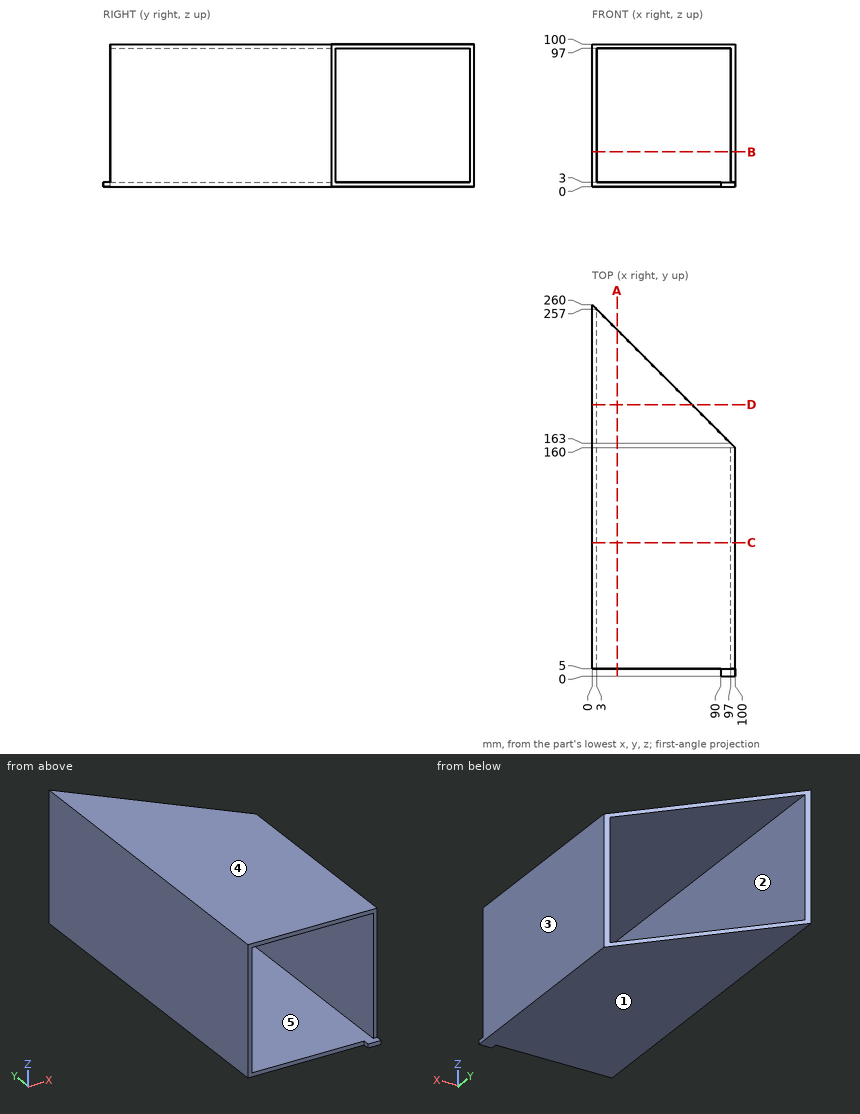
Here's the drawing with two shaded views (mm, measured from the low corner). I have some questions. A direction names the side the tool comes from. Give positions to 0.01 mm unless a question says otherwise; leave off trailing zeros. Order: outer loops, then holes, each group sorted by start corner. A loop starts at its lowest first (then second) coordinate and runs counter-clockwise, first axis right, second up.
Q1. Suppose I cut it at B-B, the plane z = 24.5. Write out the boundary of the cut face in (x, y).
Q2. Suppose I cut it at C-C, the plane y = 93.5. Write out the boundary of the cut face in (x, z), and give its area (3 significant figures).
Q3. For the marked faces 1 and 2, which set-ups out of +Z, -Z, +X, -X, +Y, -Y let a thin tool reach every point of the face, with its end or its side?
Q4. Suppose I cut it at D-D, the plane y = 190. Write out the boundary of the cut face in (x, z), and give its area (3 significant figures).
Q5. If I drill on line 1 along X through (y, z) = (90.5, 35.5); line 2 along X through (y, z) = (169, 17.5), over which ranges is the centre line in solid material (lowest first)?
Q6. Suppose I cut it at A-A, the plane x = 17.5. Write out the boundary of the cut face in (y, z), and give its area (4 significant figures).
Q7. I'm going to push flat-ended pins straight in: P1, Ø0.9, axis at y = 3, z = 2, coming from the -X side; P2, Ø2, axis at x = 31, y = 170, coming from the -Z side; P3, Ø1, axis at y = 177.5, z = 42.5, coming from the +X side. Where does each tip first touch, or does it pass through?
Q8. We'd pull the mould along Z, two halves only. Please class the marked faces 3, 4 and 5: +Z half, -Z half, draft (parallel to the pull), parting line (faces both ways), or undercut.
Solution:
1. outline: (0, 5) - (3, 5) - (3, 257) - (0, 260) - close; (97, 5) - (100, 5) - (100, 160) - (97, 163) - close
2. outline: (0, 0) - (100, 0) - (100, 100) - (0, 100) - close; hole (3, 3) - (97, 3) - (97, 97) - (3, 97) - close
2. area: 1,160 mm2
3. face 1: -Z, +X, -X, +Y, -Y
3. face 2: +Y, -Y
4. outline: (0, 0) - (70, 0) - (70, 3) - (3, 3) - (3, 97) - (70, 97) - (70, 100) - (0, 100) - close
4. area: 702 mm2
5. line 1: x = 0 to 3, 97 to 100
5. line 2: x = 0 to 3
6. outline: (5, 0) - (242.5, 0) - (242.5, 3) - (5, 3) - close; (5, 97) - (242.5, 97) - (242.5, 100) - (5, 100) - close
6. area: 1,425 mm2
7. P1: stops at x = 90
7. P2: stops at z = 0
7. P3: stops at x = 3
8. face 3: draft
8. face 4: +Z half
8. face 5: undercut
